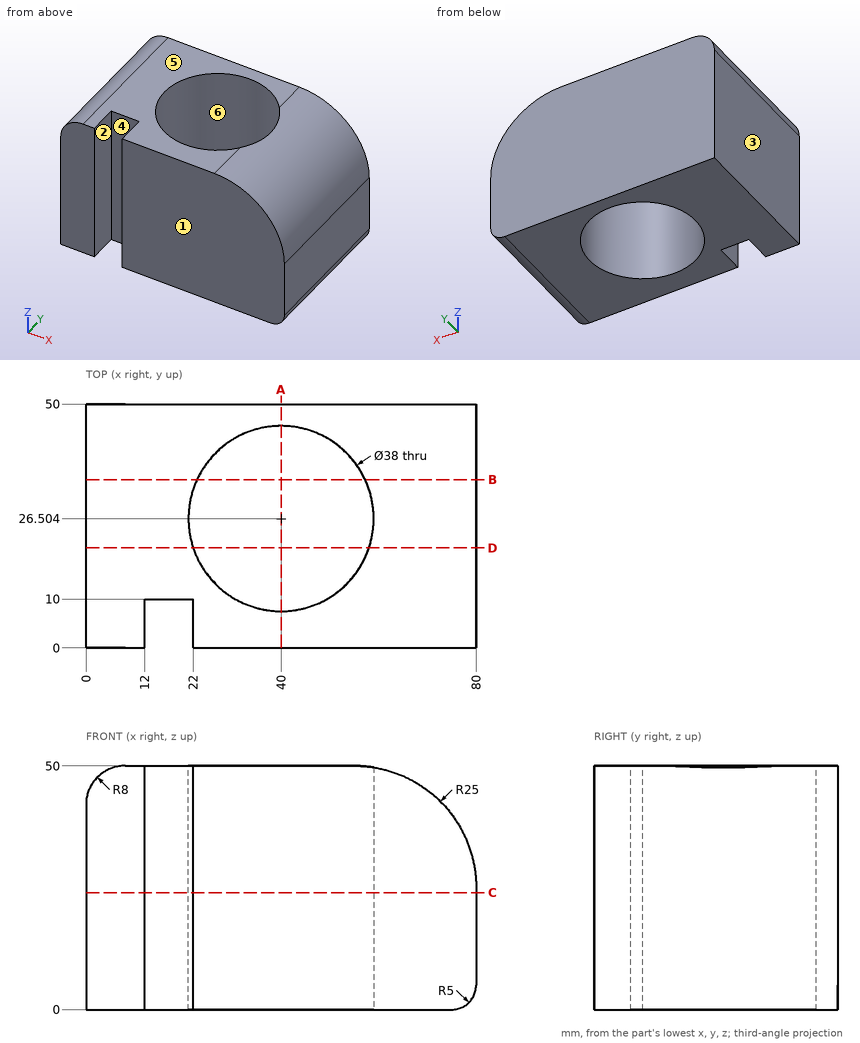
Could you check a few things on this drawing? It's one solid part, dimensions in mm from its lowest x, y, z. A direction names the side the tool comes from. Coordinates: 2 decimals unless noted, no trailing zeros. Order: outer loops, then holes, each group sorted by start corner. A loop starts at its lowest first (then second) coordinate and runs counter-clockwise, first axis right, second up. Notation, with made-up numbers: M 33.25,9.5 L 43.25,9.5 A26 cw 43.25,33.5 Z; hole C 65,57.5 d11. An arc over 180 degrees is marked long. Use a Markdown table: item, result. Add a question column.
Q1. Which directions (+Z, -Z, +X, -X, +Y, -Y) give clear straight access to the entire face, cutting with the end or side of a thin tool? Please do the marked faces 1 and 2.
Q2. I'm going to push flat-ended pins straight in: pin 1 (1.5 mm diameter, centred on x = 55.5, y = 41.5, fed in from +Z); pin 2 (3 mm diameter, centred on x = 19, z = 6, fed in from -Y); pin 3 (10 mm diameter, centred on y = 6, z = 42, fed in from +X). Where does each tip first touch, or does it pass through?
Q3. I want a section at A-A on x = 40. List the corners of the cut face in (y, z) for me, then the cut area to 3 significant figures.
Q4. I want a section at D-D on y = 20.5. List the corners of the cut face in (x, z) for me, then the cut area to 3 significant figures.
Q5. I want a section at B-B on y = 34.5. List the corners of the cut face in (x, z) for me.
Q6. I want a section at C-C on z = 24. List the corners of the cut face in (x, y) for me, then the cut area to 3 significant figures.
Q7. We'd pull the mould along X, two halves only. Please class the marked faces 3, 4, 5 and 6: pulls with the +X half, pulls with the -X half, needs draft (parallel to the pull), parting line crosses it, or undercut.
Q8. If I drill on L1, parallel to X at y = 4.5, z = 12.5; L2, parallel to Y at x = 40, z = 34; L3, parallel to Y at x = 15, z = 8.5, over which ranges is the centre line in solid material (lowest first)?
Checked values:
| question | item | result |
|---|---|---|
| 1 | face 1 | +Z, -Z, +X, -X, -Y |
| 1 | face 2 | +Z, -Z, -Y |
| 2 | pin 1 | z = 50 |
| 2 | pin 2 | y = 10 |
| 2 | pin 3 | x = 76.93 |
| 3 | outline | M 0,0 L 7.5,0 L 7.5,50 L 0,50 Z; M 45.5,0 L 50,0 L 50,50 L 45.5,50 Z |
| 3 | area | 600 mm² |
| 4 | outline | M 0,0 L 21.97,0 L 21.97,50 L 8,50 A8 ccw 0,42 Z; M 58.03,0 L 75,0 A5 ccw 80,5 L 80,25 A25 ccw 58.03,49.82 Z |
| 4 | area | 2,040 mm² |
| 5 | outline | M 0,0 L 22.76,0 L 22.76,50 L 8,50 A8 ccw 0,42 Z; M 57.24,0 L 75,0 A5 ccw 80,5 L 80,25 A25 ccw 57.24,49.9 Z |
| 6 | outline | M 0,0 L 12,0 L 12,10 L 22,10 L 22,0 L 80,0 L 80,50 L 0,50 Z; hole C 40,26.5 d38 |
| 6 | area | 2,770 mm² |
| 7 | face 3 | pulls with the -X half |
| 7 | face 4 | undercut |
| 7 | face 5 | needs draft |
| 7 | face 6 | undercut |
| 8 | L1 | 0 to 12, 22 to 80 |
| 8 | L2 | 0 to 7.5, 45.5 to 50 |
| 8 | L3 | 10 to 50 |
